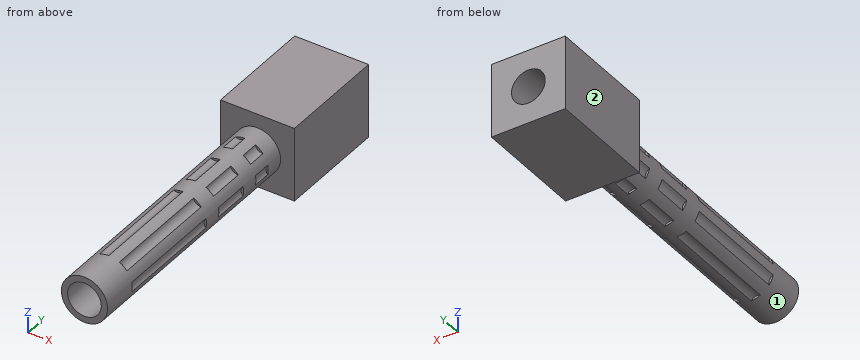
```python
from build123d import *

# Parameters (mm, degrees)
F0_W     = 25.4
F0_H     = 25.4
F0_R     = 7.9375
F0_R_2   = 5.8024107256
F1_DEPTH = 38.1
F2_DEPTH = 127
F4_START = -12.7
F3_R     = 2.4554456834
F4_DEPTH = 38.1
F5_START = -57.15
F5_DEPTH = 12.7
F6_START = -76.2
F6_DEPTH = 6.35


with BuildPart() as f1:
    # F0 (on Front) → F1 (new body)
    with BuildSketch(Plane.XZ):
        Rectangle(F0_W, F0_H)
        Circle(F0_R, mode=Mode.SUBTRACT)
        Circle(F0_R)
        Circle(F0_R_2, mode=Mode.SUBTRACT)
    extrude(amount=F1_DEPTH)

    # F0 (on Front) → F2 (join)
    with BuildSketch(Plane.XZ):
        Circle(F0_R)
        Circle(F0_R_2, mode=Mode.SUBTRACT)
    extrude(amount=F2_DEPTH)

    # F3 (on face) → F4 (cut)
    with BuildSketch(Plane.XZ.offset(127).offset(F4_START)):
        with Locations((9.5774363726, 0)):
            Circle(F3_R)
        with Locations((5.9714339063, 7.4879412775)):
            Circle(F3_R)
        with Locations((-2.1311800865, 9.3373100468)):
            Circle(F3_R)
        with Locations((-8.6289720061, 4.1554939045)):
            Circle(F3_R)
        with Locations((-8.6289720061, -4.1554939045)):
            Circle(F3_R)
        with Locations((-2.1311800865, -9.3373100468)):
            Circle(F3_R)
        with Locations((5.9714339063, -7.4879412775)):
            Circle(F3_R)
    extrude(amount=-F4_DEPTH, mode=Mode.SUBTRACT)

    # F3 (on face) → F5 (cut)
    with BuildSketch(Plane.XZ.offset(127).offset(F5_START)):
        with Locations((9.5774363726, 0)):
            Circle(F3_R)
        with Locations((5.9714339063, 7.4879412775)):
            Circle(F3_R)
        with Locations((-2.1311800865, 9.3373100468)):
            Circle(F3_R)
        with Locations((-8.6289720061, 4.1554939045)):
            Circle(F3_R)
        with Locations((-8.6289720061, -4.1554939045)):
            Circle(F3_R)
        with Locations((-2.1311800865, -9.3373100468)):
            Circle(F3_R)
        with Locations((5.9714339063, -7.4879412775)):
            Circle(F3_R)
    extrude(amount=-F5_DEPTH, mode=Mode.SUBTRACT)

    # F3 (on face) → F6 (cut)
    with BuildSketch(Plane.XZ.offset(127).offset(F6_START)):
        with Locations((9.5774363726, 0)):
            Circle(F3_R)
        with Locations((5.9714339063, 7.4879412775)):
            Circle(F3_R)
        with Locations((-2.1311800865, 9.3373100468)):
            Circle(F3_R)
        with Locations((-8.6289720061, 4.1554939045)):
            Circle(F3_R)
        with Locations((-8.6289720061, -4.1554939045)):
            Circle(F3_R)
        with Locations((-2.1311800865, -9.3373100468)):
            Circle(F3_R)
        with Locations((5.9714339063, -7.4879412775)):
            Circle(F3_R)
    extrude(amount=-F6_DEPTH, mode=Mode.SUBTRACT)


solid = f1.part
```
CAD build for the part. Positions are in the model's coordinates, mm. Face numbers are marked on the shaded views. A direction names the side the tool comes from. Give positions to 0.01 mm unless a question says otherwise; leave off trailing zeros. Write each loop counter-clockwise with the first axis right and the second up, starting at its lowest first coordinate (ties: lowest second). Pieces come first, ordered by that corner, then holes. Notation, with made-up numbers: M -6,-2 L 6,-2 A38 ccw 6,36 Z; hole C 0,18.25 d5. An arc over 180 degrees is marked long. Return JSON: item names as keys, results as strings. Group by question number.
(1) Band-saw the part on C-C (y = -100). Give the cut face in (x, z) (1 decimal).
(2) Band-saw the part on A-A (z = 0). Give the cut face in (x, y), and give its area (3 significant figures).
(3) Drill centre lines: L1, parallel to Z at x = 0, y = -84; L2, parallel to X at y = -23, z = -2; L3, parallel to Y at x = 11.75, z = 3.75. Where is each one in solid material? Low to high. Write a range as [from, to].
(4) Flat gauge pins, fed straight in: pin 1 Ø8 at (y, z) = (-71, 4) entering from +X; pin 2 Ø12 at (y, z) = (-70, 6) entering from -X; pin 3 Ø6 at (x, y) = (0, -50.5) entering from -Z. Where does each tip first touch, or does it go through?
(5) 3-axis set-ups, long thin cutter, end or side, ignore diameter. For the marked faces 1 and 2: which of +Z, -Z, +X, -X, +Y, -Y reach the whole face in a straight line?
(6) Band-saw the part on D-D (z = 11.25). Give the cut face in (x, y), and give its area (3 significant figures).
(7) Band-saw the part on B-B (y = -22.5). Give the cut face in (x, z).
Entries:
{
 "1": {"outline": "M -7.7,-1.9 A2.5 cw -6.3,-4.9 A7.9 ccw -3.3,-7.2 A2.5 cw -0.1,-7.9 A7.9 ccw 3.5,-7.1 A2.5 cw 6.1,-5 A7.9 ccw 7.8,-1.7 A2.5 cw 7.8,1.7 A7.9 ccw 6.1,5 A2.5 cw 3.5,7.1 A7.9 ccw -0.1,7.9 A2.5 cw -3.3,7.2 A7.9 ccw -6.3,4.9 A2.5 cw -7.7,1.9 A7.9 ccw Z; hole C 0,0 d11.6"},
 "2": {"outline": "M -12.7,-38.1 L -7.94,-38.1 L -7.94,-127 L -5.8,-127 L -5.8,0 L -12.7,0 Z; M 5.8,-127 L 7.94,-127 L 7.94,-114.3 L 7.12,-114.3 L 7.12,-76.2 L 7.94,-76.2 L 7.94,-69.85 L 7.12,-69.85 L 7.12,-57.15 L 7.94,-57.15 L 7.94,-50.8 L 7.12,-50.8 L 7.12,-44.45 L 7.94,-44.45 L 7.94,-38.1 L 12.7,-38.1 L 12.7,0 L 5.8,0 Z", "area": "859 mm^2"},
 "3": {"L1": "z = [-7.94, -5.8], [5.8, 7.94]", "L2": "x = [-12.7, -5.45], [5.45, 12.7]", "L3": "y = [-38.1, 0]"},
 "4": {"pin 1": "stops at x = 7.94", "pin 2": "stops at x = -7.94", "pin 3": "stops at z = -7.94"},
 "5": {"face 1": "-Y", "face 2": "+Z, -Z, -X, +Y, -Y"},
 "6": {"outline": "M -12.7,-38.1 L 12.7,-38.1 L 12.7,0 L -12.7,0 Z", "area": "968 mm^2"},
 "7": {"outline": "M -12.7,-12.7 L 12.7,-12.7 L 12.7,12.7 L -12.7,12.7 Z; hole C 0,0 d11.6"}
}
